Autodesk Inventor part; units mm, degrees
ref_plane "Work Plane1" through (0, -6, 0) normal (1, 0, 0) x (0, 0, 1)
ref_plane "YZ Plane" through (0, 0, 0) normal (1, 0, 0) x (0, 1, 0)
ref_plane "XZ Plane" through (0, 0, 0) normal (0, 1, 0) x (-1, 0, 0)
sketch "Szkic1" plane through (0, 0, 0) normal (0, 0, 1) x (1, 0, 0)
  line L0 (-6, 0) -> (6, 0) construction
  arc A0 (0.425, -11.7343) -> (-0.425, -11.7343) centre (0, -6) ccw
  line L1 (0, 20.1894) -> (0, -80.5364)
  line L2 (-48.09, 0) -> (48.09, 0)
  line L3 (-0.425, -11.7343) -> (-0.425, -15.0343)
  line L4 (-0.425, -6.5402) -> (-0.425, -13.29) construction
  line L5 (-2.7947, 1.8) -> (3.6722, 1.8) construction
  arc A1 (4.1403, -11.6229) -> (-4.1403, -11.6229) centre (0, -5.55) ccw
  arc A2 (-2.0935, -14.7986) -> (-0.425, -15.0343) centre (0, -6) ccw
  arc A3 (-3.399, -13.0862) -> (-2.0935, -14.7986) centre (-1.7, -13.1448) ccw
  arc A4 (-3.399, -13.0862) -> (-4.1403, -11.6229) centre (-5.098, -13.0275) ccw
  line L6 (0.425, -11.7343) -> (0.425, -15.0343)
  line L7 (0.425, -6.5402) -> (0.425, -13.29) construction
  arc A5 (0.425, -15.0343) -> (2.0935, -14.7986) centre (0, -6) ccw
  arc A6 (2.0935, -14.7986) -> (3.399, -13.0862) centre (1.7, -13.1448) ccw
  arc A7 (4.1403, -11.6229) -> (3.399, -13.0862) centre (5.098, -13.0275) ccw
  circle A8 centre (-1.7, -13.1448) radius 0.85
  circle A9 centre (1.7, -13.1448) radius 0.85
  dimension "d0" = 11.5
  dimension "d1" = 3.3
  dimension "d6" = 0.425
  dimension "d7" = 1.8
  dimension "d8" = 0.45
  dimension "d9" = 1.7
  dimension "d10" = 1.7
  dimension "d11" = 1.275
  dimension "d12" = 1.7
  dimension "d13" = 1.7
  dimension "d14" = 6
extrude "Bryła" add sketch "Szkic1" along normal blind 1
ref_plane "Work Plane1" through (0, -6, 0) normal (1, 0, 0) x (0, 0, 1)
equation "\"d0\" = ND"
equation "\"d1\" = SRB2"
equation "\"d6\" = 0.25 * SD5"
equation "\"d7\" = SRB1"
equation "\"d8\" = 0.25 * SRB1"
equation "\"d9\" = SD5"
equation "\"d10\" = SD5"
equation "\"d11\" = 0.75 * SD5"
equation "\"d12\" = SD5"
equation "\"d13\" = SD5"
equation "\"d14\" = 0.5 * WD"
equation "\"d2\" = SD"
equation "\"WD\" = WDMIN"
equation "\"SD\" = 1"
equation "\"SRB1\" = 1.8"
equation "\"ND\" = 11.5"
equation "\"SRB2\" = 3.3"
equation "\"SD5\" = 1.7"
equation "\"WDMIN\" = 12"
equation "\"SD3\" = 11"
equation "\"WDMAX\" = 13"
properties part number "DIN 471 - 12 x 1" material "Stal, miękka"
Can you work these out from the model? Positions are in its coordinate system, mm. A direction names the side the tool comes from. Coordinates: 2 decimals unless noted, no trailing zeros. Order: outer loops, then holes, each group sorted by start corner. A loop starts at its lowest first (then second) coordinate and runs counter-clockwise, first axis right, second up. Notation, with made-up numbers: (42, -26) - (62, -26) arc R21 cw to (62, 12) - close; hole circle Ø4 at (68, 84). An arc over 180 degrees is marked (long way). Answer in a Markdown table with one row per item.
1. Suppose I cut it at D-D (x = -3). Please give me the cut outline in (y, z).
Reply:
| item | result |
|---|---|
| outline | (-14.24, 0) - (-10.91, 0) - (-10.91, 1) - (-14.24, 1) - close; (-1.09, 0) - (1.16, 0) - (1.16, 1) - (-1.09, 1) - close |
2. If we mould it in two halves opening along X, with no side actions, what happens to faces 1 (the cylindrical face through (-1.811, -13.988, 0.493)), 2 (the cylindrical face through (1.276, -14.954, 0.493)), 3 (the cylindrical face through (-1.253, -14.957, 0.493)), 4 (the cylindrical face through (1.589, -13.988, 0.493))? For each: pulls with the +X half, pulls with the -X half, needs draft (parallel to the pull), parting line crosses it, or undercut.
Reply:
| item | result |
|---|---|
| face 1 | undercut |
| face 2 | pulls with the +X half |
| face 3 | pulls with the -X half |
| face 4 | undercut |
3. For pin 1 (0.5 mm diameter, centred on y = -14, z = 0.5, fed in from -X), with a flat end and sliding along its axis, tell me the tip position at first contact or that it passes through.
Reply:
| item | result |
|---|---|
| pin 1 | stops at x = -3.29 |
4. For faces 5 (the flat face through (0.425, -13.4, 0.5)), 6 (the cylindrical face through (-0.262, 1.795, 0.493)), which set-ups out of +Z, -Z, +X, -X, +Y, -Y let a thin tool reach every point of the face, with its end or its side?
Reply:
| item | result |
|---|---|
| face 5 | +Z, -Z, -Y |
| face 6 | +Z, -Z |
5. Suppose I cut it at B-B (x = -1.25). Please give me the cut outline in (y, z), and give its area (3 significant figures).
Reply:
| item | result |
|---|---|
| outline | (-14.96, 0) - (-13.87, 0) - (-13.87, 1) - (-14.96, 1) - close; (-12.42, 0) - (-11.61, 0) - (-11.61, 1) - (-12.42, 1) - close; (-0.39, 0) - (1.69, 0) - (1.69, 1) - (-0.39, 1) - close |
| area | 3.98 mm^2 |
6. If I drill on line 1 along Y through (x, z) = (1.5, 0.7); line 2 along Y through (x, z) = (-1, 0.6); line 3 along Y through (x, z) = (0, 0.35), over which ranges is the centre line in solid material (lowest first)?
Reply:
| item | result |
|---|---|
| line 1 | y = -14.92 to -13.97, -12.32 to -11.55, -0.45 to 1.65 |
| line 2 | y = -14.99 to -13.63, -12.66 to -11.66, -0.34 to 1.73 |
| line 3 | y = -0.25 to 1.8 |
7. Suppose I cut it at C-C (z = 0.4). Give the number of separate pieces and of enclosed holes in the cut face, and give its area (3 significant figures).
Reply:
| item | result |
|---|---|
| separate pieces | 1 |
| enclosed holes | 2 |
| area | 73.1 mm^2 |
8. Suppose I cut it at A-A (y = -8.25). Please give me the cut outline in (x, z).
Reply:
| item | result |
|---|---|
| outline | (-6.84, 0) - (-5.29, 0) - (-5.29, 1) - (-6.84, 1) - close; (5.29, 0) - (6.84, 0) - (6.84, 1) - (5.29, 1) - close |
